Verification items for the finished model (mm, model axes). Give positions to 0.01 mm unless a question says otherwise; leave off trailing zeros. Write each loop counter-clockwise with the first axis right and the second up, starting at its lowest first coordinate (ties: lowest second). Pieces come first, ordered by that corner, then holes.
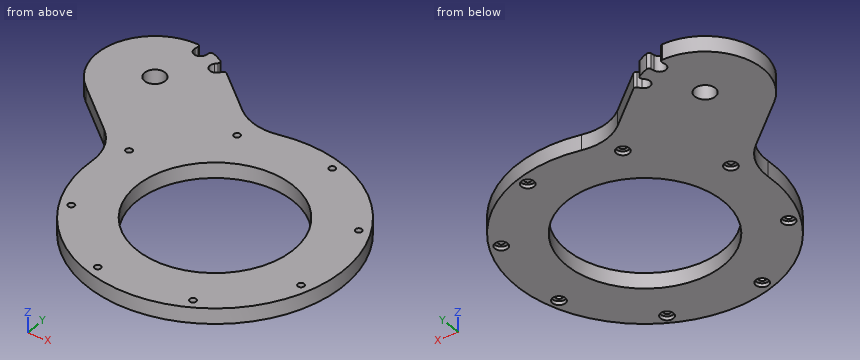
from build123d import *

# Parameters (mm, degrees)
EXTRUDE_2_DEPTH      = 1
EXTRUDE_2_DEPTH_BACK = 5
SKETCH_1_R           = 4
SKETCH_2_R           = 1.25
SKETCH_2_R_2         = 30.5
CUT_EXTRUDE_1_DEPTH  = 10
SKETCH_3_R           = 2.5
CUT_EXTRUDE_2_DEPTH  = 1.5


with BuildPart() as part:
    # 草图1 → 凸台-拉伸2 (new, two sides: drawn at the far end of the back side and taken through both)
    with BuildSketch(Plane.XY.offset(-EXTRUDE_2_DEPTH_BACK)):
        with BuildLine():
            Line((-28.145811083, 52.988803709), (-44.139678681, 66.409252111))
            ThreePointArc((-44.139678681, 66.409252111), (-44.869622033, 66.639402366), (-45.548510733, 66.285995278))
            Line((-45.548510733, 66.285995278), (-46.512692148, 65.136928613))
            ThreePointArc((-46.512692148, 65.136928613), (-50.03477228, 64.82878653), (-50.342914364, 68.350866662))
            Line((-50.342914364, 68.350866662), (-49.563082227, 69.280234412))
            ThreePointArc((-49.563082227, 69.280234412), (-49.343377533, 70.09124401), (-49.819618355, 70.783487754))
            ThreePointArc((-49.819618355, 70.783487754), (-51.77464456, 71.814933983), (-53.821444834, 72.649570088))
            ThreePointArc((-53.821444834, 72.649570088), (-54.657856007, 72.569426022), (-55.137901948, 71.87981554))
            Line((-55.137901948, 71.87981554), (-55.348572514, 70.685043391))
            ThreePointArc((-55.348572514, 70.685043391), (-58.24471234, 68.657144453), (-60.272611279, 71.553284279))
            Line((-60.272611279, 71.553284279), (-60.061940713, 72.748056429))
            ThreePointArc((-60.061940713, 72.748056429), (-60.277175665, 73.560263691), (-61.035734188, 73.921643947))
            ThreePointArc((-61.035734188, 73.921643947), (-82.383938211, 59.234784971), (-75.746276667, 34.187008805))
            Line((-75.746276667, 34.187008805), (-57.071253519, 18.516803768))
            ThreePointArc((-57.071253519, 18.516803768), (-51.612575359, 11.232185237), (-49.947861223, 2.282796361))
            ThreePointArc((-49.947861223, 2.282796361), (38.302222156, -32.139380484), (-10.921470635, 48.792637551))
            ThreePointArc((-10.921470635, 48.792637551), (-20.02397276, 48.878015869), (-28.145811083, 52.988803709))
        make_face()
        with Locations((-61.28355545, 51.423008775)):
            Circle(SKETCH_1_R, mode=Mode.SUBTRACT)
    extrude(amount=EXTRUDE_2_DEPTH + EXTRUDE_2_DEPTH_BACK)

    # 草图2 → 切除-拉伸1 (cut)
    with BuildSketch(Plane.XY.offset(1)):
        with Locations((-21.240436209, 40.802498326)):
            Circle(SKETCH_2_R)
        with Locations((13.832466777, 43.870979734)):
            Circle(SKETCH_2_R)
        with Locations((40.802498326, 21.240436209)):
            Circle(SKETCH_2_R)
        with Locations((43.870979734, -13.832466777)):
            Circle(SKETCH_2_R)
        with Locations((21.240436209, -40.802498326)):
            Circle(SKETCH_2_R)
        with Locations((-13.832466777, -43.870979734)):
            Circle(SKETCH_2_R)
        with Locations((-40.802498326, -21.240436209)):
            Circle(SKETCH_2_R)
        with Locations((-43.870979734, 13.832466777)):
            Circle(SKETCH_2_R)
        Circle(SKETCH_2_R_2)
    extrude(amount=-CUT_EXTRUDE_1_DEPTH, mode=Mode.SUBTRACT)

    # 草图3 → 切除-拉伸2 (cut)
    with BuildSketch(Plane(origin=(0, 0, -5), x_dir=(-1, 0, 0), z_dir=(0, 0, -1))):
        with Locations((-13.832466777, 43.870979734)):
            Circle(SKETCH_3_R)
        with Locations((21.240436209, 40.802498326)):
            Circle(SKETCH_3_R)
        with Locations((43.870979734, 13.832466777)):
            Circle(SKETCH_3_R)
        with Locations((40.802498326, -21.240436209)):
            Circle(SKETCH_3_R)
        with Locations((13.832466777, -43.870979734)):
            Circle(SKETCH_3_R)
        with Locations((-21.240436209, -40.802498326)):
            Circle(SKETCH_3_R)
        with Locations((-43.870979734, -13.832466777)):
            Circle(SKETCH_3_R)
        with Locations((-40.802498326, 21.240436209)):
            Circle(SKETCH_3_R)
    extrude(amount=-CUT_EXTRUDE_2_DEPTH, mode=Mode.SUBTRACT)


solid = part.part
Item 1: Sectioned sample at A-A on y = 0. Record the cut outline in (x, z), then the cut area to 3 significant figures.
Answer key:
outline: (-50, -5) - (-30.5, -5) - (-30.5, 1) - (-50, 1) - close; (30.5, -5) - (50, -5) - (50, 1) - (30.5, 1) - close
area: 234 mm2
Item 2: Sectioned sample at D-D on y = -34. Record the cut outline in (x, z).
Answer key:
outline: (-36.66, -5) - (36.66, -5) - (36.66, 1) - (-36.66, 1) - close
Item 3: Depth check by flat-ended pin: pin 1 (4.5 mm diameter, centred on x = 43.87, y = -13.83, fed in from -Z); pin 2 (6.5 mm diameter, centred on x = -61.28, y = 51.42, fed in from -Z); pin 3 (1.5 mm diameter, centred on y = -15.5, z = -4.5, fed in from +X); pin 4 (1.5 mm diameter, centred on x = -30, z = 0.5, fed in from -Y). Enter the tip coordinate at first touch or a pass-through.
Answer key:
pin 1: stops at z = -3.5
pin 2: passes through
pin 3: stops at x = 47.77
pin 4: stops at y = -40.55
Item 4: Sectioned sample at C-C on z = -2.3. State how many separate pieces and enclosed holes the cut face has, then the cut area to 3 significant figures.
Answer key:
separate pieces: 1
enclosed holes: 10
area: 7,050 mm2
Item 5: Scan lines: line 1 along X through (y, z) = (0.5, -0.5); line 2 along X through (y, z) = (-15.5, -4.45); line 3 along X through (y, z) = (3.5, -2.05). Record each from-to range of solid material in increasing order.
Answer key:
line 1: x = -50 to -30.5, 30.5 to 50
line 2: x = -47.54 to -26.27, 26.27 to 42.01, 45.73 to 47.54
line 3: x = -49.93 to -30.3, 30.3 to 49.88
